For this review, use the dimensioned drawing (mm, ordinates from the lowest corner) and the shaded views. A direction names the side the tool comes from. Round coordinates to 2 decimals unless told otherwise and drop trailing zeros. Loops run counter-clockwise (first coordinate to the right, second up) from the corner with the lowest first, then second, coordinate; pieces in that order, holes last. Notation, with made-up numbers: M -23,89.5 L -5,89.5 A34 ccw -5,122.5 Z; hole C -31,71 d6. An arc over 180 degrees is marked long. Answer as a JSON object with one key per item and string values. Group by question number.
Item 1: Consider section D-D (z = 26). Give the boundary of the cut face in (x, y).
Item 2: To check wall thickness, follow line 1 (Z direction, x = 25, y = 5.5); line 2 (Z direction, x = 25, y = 10.6); line 3 (X direction, y = 4.75, z = 37). State the ranges of each line that lie inside material, in increasing order.
Item 3: Tool access review of the marked faces 1 and 2: name each direction out of +Z, -Z, +X, -X, +Y, -Y from which nothing blocks a thin tool from reaching the whole face with its end or side.
Item 4: Consider section B-B (y = 7). Give the boundary of the cut face in (x, z).
Item 5: Consider section A-A (x = 25). Give the boundary of the cut face in (y, z), and give its area (3 significant figures).
Item 6: Insertion check: P1, Ø1, axis at y = 4.5, z = 42, coming from the +X side; P2, Ø24, axis at x = 12.01, z = 32.5, coming from the -Y side; P3, Ø4, axis at y = 2.5, z = 34, coming from the -X side; P4, Ø12, axis at x = 37.99, z = 32.5, coming from the -Y side. Each pin has a flat end and moves straight along its axis. Give the tip position at first contact, or say it passes through.
Item 7: The part is to be moulded in two halves that separate along Z. For the marked faces 3 and 4, say which applies: +Z half, -Z half, draft (parallel to the pull), parting line (faces both ways), or undercut.
Item 8: Consider section C-C (z = 10). Give the boundary of the cut face in (x, y), and give its area (3 significant figures).
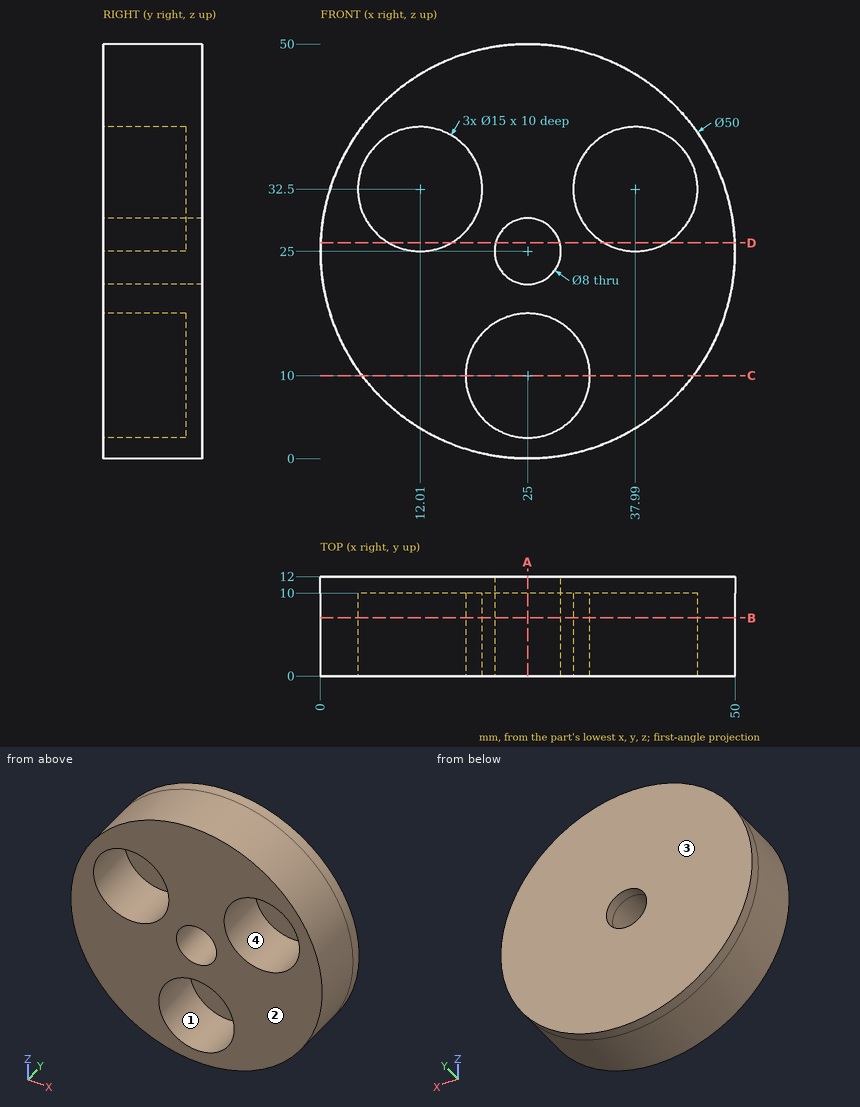
Geometry results:
{
 "1": {"outline": "M 0.02,0 L 8.27,0 L 8.27,10 L 15.75,10 L 15.75,0 L 21.13,0 L 21.13,12 L 0.02,12 Z; M 28.87,0 L 34.25,0 L 34.25,10 L 41.73,10 L 41.73,0 L 49.98,0 L 49.98,12 L 28.87,12 Z"},
 "2": {"line 1": "z = 0 to 2.5, 17.5 to 21, 29 to 50", "line 2": "z = 0 to 21, 29 to 50", "line 3": "x = 3.07 to 6.01, 18.01 to 31.99, 43.99 to 46.93"},
 "3": {"face 1": "-Y", "face 2": "+Z, -Z, +X, -X, -Y"},
 "4": {"outline": "C 25,25 d50; hole C 12.01,32.5 d15; hole C 25,10 d15; hole C 25,25 d8; hole C 37.99,32.5 d15"},
 "5": {"outline": "M 0,0 L 12,0 L 12,21 L 0,21 L 0,17.5 L 10,17.5 L 10,2.5 L 0,2.5 Z; M 0,29 L 12,29 L 12,50 L 0,50 Z", "area": "354 mm^2"},
 "6": {"P1": "stops at x = 43.78", "P2": "stops at y = 0", "P3": "stops at x = 1", "P4": "stops at y = 10"},
 "7": {"face 3": "draft", "face 4": "undercut"},
 "8": {"outline": "M 5,0 L 17.5,0 L 17.5,10 L 32.5,10 L 32.5,0 L 45,0 L 45,12 L 5,12 Z", "area": "330 mm^2"}
}
